from build123d import *

# Parameters (mm, degrees)
F0_W     = 42.3
F0_H     = 42.3
F1_DEPTH = 48
F2_SIZE  = 4.445
F4_DEPTH = 4.8768


with BuildPart() as f1:
    # F0 (on Top) → F1 (new body)
    with BuildSketch(Plane.XY):
        Rectangle(F0_W, F0_H)
    extrude(amount=F1_DEPTH)

    # F2
    f2_edges = [f1.edges().sort_by_distance(p)[0] for p in [
        (21.15, 21.15, 24),
        (-21.15, 21.15, 24),
        (-21.15, -21.15, 24),
        (21.15, -21.15, 24),
    ]]
    chamfer(f2_edges, length=F2_SIZE)

    # F3 (on face) → F4 (join)
    with BuildSketch(Plane(origin=(0, 0, 0), x_dir=(1, 0, 0), z_dir=(0, 0, -1))):
        Polygon((-16.315722, -20.2102), (16.315722, -20.2102), (20.2102, -16.315722), (20.2102, 16.315722), (16.315722, 20.2102), (-16.315722, 20.2102), (-20.2102, 16.315722), (-20.2102, -16.315722), align=None)
    extrude(amount=F4_DEPTH)


solid = f1.part
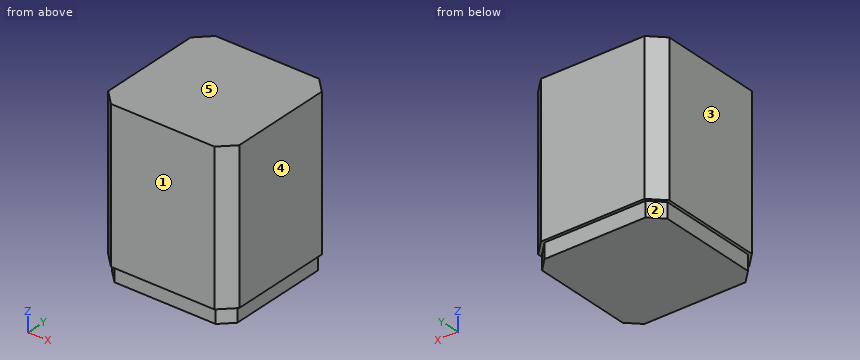
Design review of the part built by this model. Coordinates are the model's own, in mm. Face numbers are marked on the shaded views. A direction names the side the tool comes from. Round coordinates to 2 decimals unless told otherwise and drop trailing zeros. Loops run counter-clockwise (first coordinate to the right, second up) from the corner with the lowest first, then second, coordinate; pieces in that order, holes last. Notation, with made-up numbers: M 71,81.5 L 85,81.5 A22 ccw 85,109.5 Z; hole C 66.5,-19.75 d2. An arc over 180 degrees is marked long. Answer as a JSON object with one key per item and string values.
Item 1: The part is to be moulded in two halves that separate along X. For the marked faces 3, 4 and 5, say which applies: pulls with the +X half, pulls with the -X half, needs draft (parallel to the pull), parting line crosses it, or undercut.
Answer sheet:
{"face 3": "pulls with the -X half", "face 4": "pulls with the +X half", "face 5": "needs draft"}
Item 2: We need section B-B on x = -17.5. Give the boundary of the cut face in (y, z) (3 decimals), and give its area (3 significant figures).
Answer sheet:
{"outline": "M -20.355,0 L -19.026,0 L -19.026,-4.877 L 19.026,-4.877 L 19.026,0 L 20.355,0 L 20.355,48 L -20.355,48 Z", "area": "2,140 mm^2"}
Item 3: Clearance check with flat-ended pins moving along their axes: P1, Ø10, axis at y = -17, z = 16.5, coming from the +X side; P2, Ø1.5, axis at x = 6, z = -2, coming from the -Y side; P3, Ø1.5, axis at x = 1, z = -2.5, coming from the +Y side; P4, Ø1.5, axis at y = 1.5, z = -3, coming from the +X side. State where each tip first meets the part, or that it passes through.
Answer sheet:
{"P1": "stops at x = 21.15", "P2": "stops at y = -20.21", "P3": "stops at y = 20.21", "P4": "stops at x = 20.21"}
Item 4: Machinability: for the marked faces 1 and 2, which of the approach directions +Z, -Z, +X, -X, +Y, -Y give a long, thin tool a straight path to every point of the face, cutting with its end or side? Answer none if there is none.
Answer sheet:
{"face 1": "+Z, -Z, +X, -X, -Y", "face 2": "-Z, -X, +Y"}
Item 5: Wall thickness on L1, parallel to Y at x = -17, z = 4 (3 decimals); L2, parallel to X at y = -17.5, z = 13 (3 decimals); L3, parallel to X at y = -18.5, z = 7 (3 decimals): over which ranges is each line inside the solid? List them lowest first. Write a range as from..to.
Answer sheet:
{"L1": "y = -20.855..20.855", "L2": "x = -20.355..20.355", "L3": "x = -19.355..19.355"}
Item 6: We need section A-A on z = 31.5. Give the boundary of the cut face in (x, y) (3 decimals), and give its area (3 significant figures).
Answer sheet:
{"outline": "M -21.15,-16.705 L -16.705,-21.15 L 16.705,-21.15 L 21.15,-16.705 L 21.15,16.705 L 16.705,21.15 L -16.705,21.15 L -21.15,16.705 Z", "area": "1,750 mm^2"}
